Design review of the part built by this model. Coordinates are the model's own, in mm. Face numbers are marked on the shaded views. A direction names the side the tool comes from. Give positions to 0.01 mm unless a question says otherwise; leave off trailing zeros. Write each loop counter-clockwise with the first axis right and the second up, starting at its lowest first coordinate (ties: lowest second). Pieces come first, ordered by that corner, then holes. Notation, with made-up numbers: (-22, 55) -> (-3, 55) arc R15 cw to (-3, 80) -> close; hole circle Ø5 at (20.25, 43). An arc over 180 degrees is marked (long way). Put each result on its own line as item: value. Start each with the question number.
from build123d import *

# Parameters (mm, degrees)
SKETCH_2_W         = 90
SKETCH_2_H         = 90
EXTRUDE_1_DEPTH    = 7
SKETCH_3_R         = 44.5
EXTRUDE_2_DEPTH    = 145
SKETCH_4_W         = 90
SKETCH_4_H         = 90
EXTRUDE_3_DEPTH    = 65
SKETCH_6_R         = 7.5
EXTRUDE_4_DEPTH    = 38
HOLE_WIZARD_M6_1_D = 5


with BuildPart() as part:
    # 草图2 → 凸台-拉伸1 (new body)
    with BuildSketch(Plane.XY):
        Rectangle(SKETCH_2_W, SKETCH_2_H)
    extrude(amount=EXTRUDE_1_DEPTH)

    # 草图3 → 凸台-拉伸2 (add)
    with BuildSketch(Plane.XY.offset(7)):
        Circle(SKETCH_3_R)
    extrude(amount=EXTRUDE_2_DEPTH)

    # 草图4 → 凸台-拉伸3 (add)
    with BuildSketch(Plane(origin=(0, 0, 0), x_dir=(-1, 0, 0), z_dir=(0, 0, -1))):
        Rectangle(SKETCH_4_W, SKETCH_4_H)
    extrude(amount=EXTRUDE_3_DEPTH)

    # 草图6 → 凸台-拉伸4 (add)
    with BuildSketch(Plane(origin=(0, 0, -65), x_dir=(-1, 0, 0), z_dir=(0, 0, -1))):
        with Locations((0, 18)):
            Circle(SKETCH_6_R)
    extrude(amount=EXTRUDE_4_DEPTH)

    # M6 螺纹孔1 (through all)
    with Locations(Plane(origin=(36.769552622, 36.769552622, -65), x_dir=(-1, 0, 0), z_dir=(0, 0, -1))):
        with Locations((0, 0), (73.539105244, 0), (73.539105244, -73.539105244), (0, -73.539105244)):
            Hole(HOLE_WIZARD_M6_1_D / 2)


solid = part.part
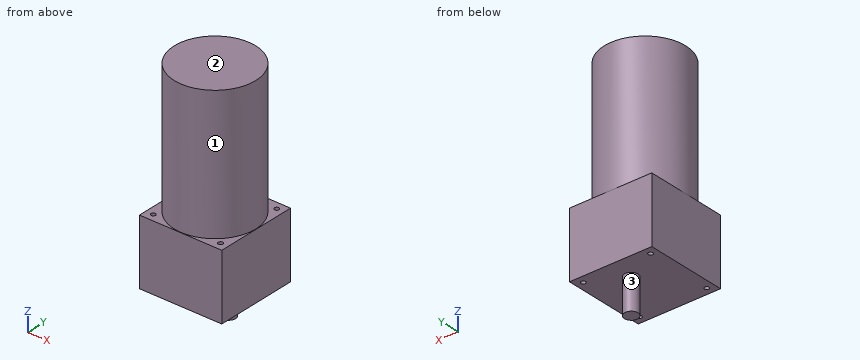
Q1. Take a section at A-A on y = 0. Give the boundary of the cut face in (x, z).
Q2. For pin 1 (6 mm diameter, centred on x = -36.77, y = 36.77, fed in from -Z); pin 2 (5 mm diameter, centred on y = 34, z = 57, fed in from -X); pin 3 (6 mm diameter, centred on x = 36.77, y = 36.77, fed in from +Z), all flat-tipped, find the tip position at first contact; note any pin that passes through.
Q3. Take a section at B-B on x = 0. Give the boundary of the cut face in (y, z).
Q4. Machinability: for the marked faces 1, 2 and 3, which of the approach directions +Z, -Z, +X, -X, +Y, -Y give a long, thin tool a straight path to every point of the face, cutting with its end or side? Answer none if there is none.
Q5. To check wall thickness, follow probe 1 along X at (y, z) = (35.5, -18); probe 2 along Z at (x, y) = (32, -9); probe 3 along Z at (x, y) = (25.5, 37). State the ranges of each line that lie inside material, in increasing order. Write a range as from..to.
Q6. Take a section at D-D on y = 29. Give the boundary of the cut face in (x, z), then the cut area to 3 significant figures.
Q7. Take a section at C-C on z = 127. Give the boundary of the cut face in (x, y), then the cut area to 3 significant figures.
Result:
1. outline: (-45, -65) -> (45, -65) -> (45, 7) -> (44.5, 7) -> (44.5, 152) -> (-44.5, 152) -> (-44.5, 7) -> (-45, 7) -> close
2. pin 1: stops at z = -65
2. pin 2: stops at x = -31.43
2. pin 3: stops at z = 7
3. outline: (-45, -65) -> (10.5, -65) -> (10.5, -103) -> (25.5, -103) -> (25.5, -65) -> (45, -65) -> (45, 7) -> (44.5, 7) -> (44.5, 152) -> (-44.5, 152) -> (-44.5, 7) -> (-45, 7) -> close
4. face 1: +Z
4. face 2: +Z, +X, -X, +Y, -Y
4. face 3: -Z
5. probe 1: x = -45..-38.92, -34.62..34.62, 38.92..45
5. probe 2: z = -65..152
5. probe 3: z = -65..7
6. outline: (-45, -65) -> (45, -65) -> (45, 7) -> (33.75, 7) -> (33.75, 152) -> (-33.75, 152) -> (-33.75, 7) -> (-45, 7) -> close
6. area: 16,300 mm^2
7. outline: circle Ø89 at (0, 0)
7. area: 6,220 mm^2
